Model file for the job. Use its own axes, mm. Coordinates: 2 decimals unless noted, no trailing zeros. Order: outer loops, then holes, each group sorted by start corner. A loop starts at its lowest first (then second) coordinate and runs counter-clockwise, first axis right, second up.
Autodesk Fusion 360 part; units mm, degrees
sketch "Sketch1" plane through (0, 0, 0) normal (0, 0, 1) x (1, 0, 0)
  circle A0 centre (0, 0) radius 30
  line L0 (10, 150) -> (-10, 150)
  line L1 (-10, 150) -> (-10, -150)
  line L2 (-10, -150) -> (10, -150)
  line L3 (10, -150) -> (10, 150)
  line L4 (10, 150) -> (-10, -150) construction
  line L5 (-10, 150) -> (10, -150) construction
  dimension "d1" = 60
  dimension "d3" = 20
  dimension "d4" = 300
extrude "Extrude1" add sketch "Sketch1" along normal blind 5
sketch "Sketch2" plane through (0, 0, 5) normal (0, 0, 1) x (-1, 0, 0)
  line L0 (-10, 150) -> (-10, 28.2843)
  arc A0 (-10, 28.2843) -> (-10, -28.2843) centre (0, 0) ccw
  line L1 (-10, -28.2843) -> (-10, -150)
  line L2 (-10, -150) -> (10, -150)
  line L3 (10, -150) -> (10, -28.2843)
  arc A1 (10, -28.2843) -> (10, 28.2843) centre (0, 0) ccw
  line L4 (10, 28.2843) -> (10, 150)
  line L5 (10, 150) -> (-10, 150)
  line L6 (30, 0) -> (-30, 0) construction
  line L7 (0, -18) -> (0, 18) construction
  point P0 (0, -140)
  point P1 (0, -110)
  point P2 (0, 140)
  point P3 (0, 110)
  point P4 (0, -18)
  point P5 (0, 18)
  dimension "d8" = 30
  dimension "d9" = 10
  dimension "d16" = 36
hole "Hole1" at (0, 0, 5) direction (0, 0, -1) diameter 8.4 end up to surface (5 mm away)
hole "Hole2" at (0, 140, 5) at (0, 110, 5) at (0, -110, 5) at (0, -140, 5) direction (0, 0, -1) diameter 3.2 end up to surface (5 mm away) countersink diameter 5.6 countersink angle 90
hole "Hole3" at (0, 18, 5) at (0, -18, 5) direction (0, 0, -1) diameter 1.8 end up to surface (5 mm away)
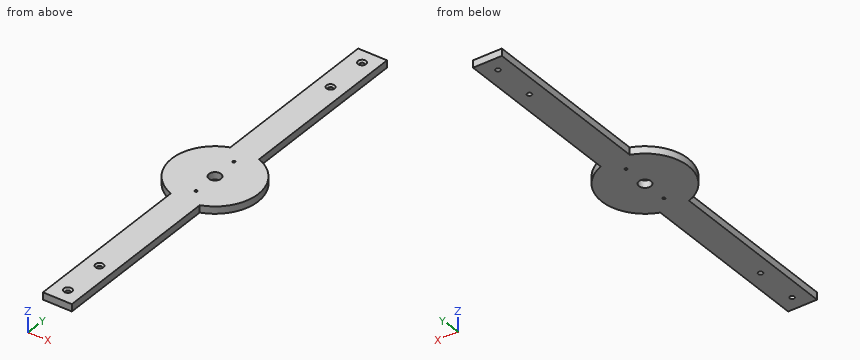
Q1. Drop flat-ended pins along their axis: P1, Ø2.5, axis at y = 95.5, z = 3, coming from the +X side; P2, Ø2, axis at x = 15, z = 3, coming from the -Y side; P3, Ø5, axis at x = 0, y = 140, coming from the +Z side. Give the stop position or say it passes through.
Established:
P1: stops at x = 10
P2: stops at y = -26.53
P3: stops at z = 4.7
Q2. Cut at B-B, the plane y = -96. List the corners of the cut face in (x, z).
Established:
outline: (-10, 0) - (10, 0) - (10, 5) - (-10, 5) - close
Q3. Cut at A-A, the plane z = 1.8. List the corners of the cut face in (x, y).
Established:
outline: (-10, -150) - (10, -150) - (10, -28.28) arc R30 ccw to (10, 28.28) - (10, 150) - (-10, 150) - (-10, 28.28) arc R30 ccw to (-10, -28.28) - close; hole circle Ø8.4 at (0, 0); hole circle Ø3.2 at (0, -140); hole circle Ø3.2 at (0, -110); hole circle Ø3.2 at (0, 110); hole circle Ø3.2 at (0, 140); hole circle Ø1.8 at (0, -18); hole circle Ø1.8 at (0, 18)
Q4. Cut at C-C, the plane x = 19. List the corners of the cut face in (y, z).
Established:
outline: (-23.22, 0) - (23.22, 0) - (23.22, 5) - (-23.22, 5) - close
Q5. Probe line 1 (X direction, y = 0, z = 3.7); line 2 (X direction, y = 110, z = 1); line 3 (X direction, y = 38, z = 3.95). List the from-to ranges inside material, lowest first.
Established:
line 1: x = -30 to -4.2, 4.2 to 30
line 2: x = -10 to -1.6, 1.6 to 10
line 3: x = -10 to 10
